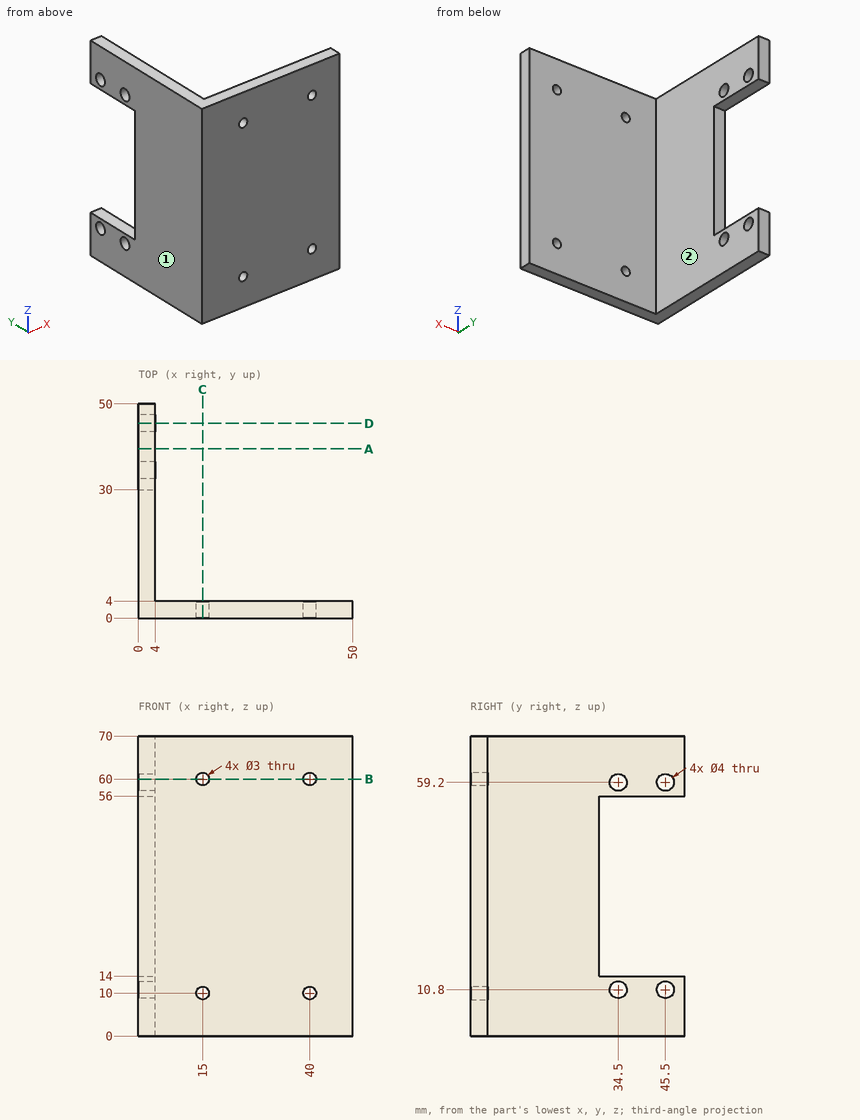
The figure shows three views and two pictorial views of one solid part (mm, origin at its lowest corner). Answer the questions. A direction names the side the tool comes from. Round coordinates to 2 decimals unless told otherwise and drop trailing zeros. Loops run counter-clockwise (first coordinate to the right, second up) from the corner with the lowest first, then second, coordinate; pieces in that order, holes last. Notation, with made-up numbers: (-12, -20.5) - (38, -20.5) arc R18 ccw to (38, 9.5) - close; hole circle Ø4 at (0, -11.75). An arc over 180 degrees is marked (long way). Use one line per item in the form item = value. Start each with the question number.
(1) Find section D-D on y = 45.5. Determine the outline of the cut face in (x, z).
(2) Find section C-C on x = 15. Determine the outline of the cut face in (y, z), and give its area (3 significant figures).
(3) Find section A-A on y = 39.5. Determine the outline of the cut face in (x, z).
(4) Find section B-B on z = 60. Determine the outline of the cut face in (x, y), and give its area (3 significant figures).
(5) Which of the six approach directions +Z, -Z, +X, -X, +Y, -Y give full straight-line access (tool end or side, diameter ignored) to the marked faces 1 and 2?
(6) Flat-ended cylindrical pins translate along their axes: P1, Ø8, axis at x = 27.5, z = 39.5, coming from the +Y side; P2, Ø3, axis at x = 2.5, z = 44.5, coming from the +Y side; P3, Ø2.5, axis at x = 15, z = 60, coming from the -Y side; P4, Ø10, axis at y = 28.5, z = 24.5, coming from the +X side. Find the tip coordinate at first contact, or state that the pin passes through.
(7) Consider line 1 (Y direction, x = 1, z = 59); line 2 (X direction, y = 1.9, z = 60); line 3 (Z direction, x = 1, y = 45). Determine where each line is inside the solid, lowest interval first.
Answer list:
q1.outline = (0, 0) - (4, 0) - (4, 8.8) - (0, 8.8) - close; (0, 12.8) - (4, 12.8) - (4, 14) - (0, 14) - close; (0, 56) - (4, 56) - (4, 57.2) - (0, 57.2) - close; (0, 61.2) - (4, 61.2) - (4, 70) - (0, 70) - close
q2.outline = (0, 0) - (4, 0) - (4, 8.5) - (0, 8.5) - close; (0, 11.5) - (4, 11.5) - (4, 58.5) - (0, 58.5) - close; (0, 61.5) - (4, 61.5) - (4, 70) - (0, 70) - close
q2.area = 256 mm^2
q3.outline = (0, 0) - (4, 0) - (4, 14) - (0, 14) - close; (0, 56) - (4, 56) - (4, 70) - (0, 70) - close
q4.outline = (0, 0) - (13.5, 0) - (13.5, 4) - (4, 4) - (4, 32.67) - (0, 32.67) - close; (0, 36.33) - (4, 36.33) - (4, 43.67) - (0, 43.67) - close; (0, 47.33) - (4, 47.33) - (4, 50) - (0, 50) - close; (16.5, 0) - (38.5, 0) - (38.5, 4) - (16.5, 4) - close; (41.5, 0) - (50, 0) - (50, 4) - (41.5, 4) - close
q4.area = 331 mm^2
q5.face_1 = +Z, -Z, -X, +Y, -Y
q5.face_2 = +Z, -Z, +X, +Y
q6.P1 = 4
q6.P2 = 30
q6.P3 = through
q6.P4 = 4
q7.line_1 = 0 to 32.51, 36.49 to 43.51, 47.49 to 50
q7.line_2 = 0 to 13.5, 16.5 to 38.5, 41.5 to 50
q7.line_3 = 0 to 8.86, 12.74 to 14, 56 to 57.26, 61.14 to 70
